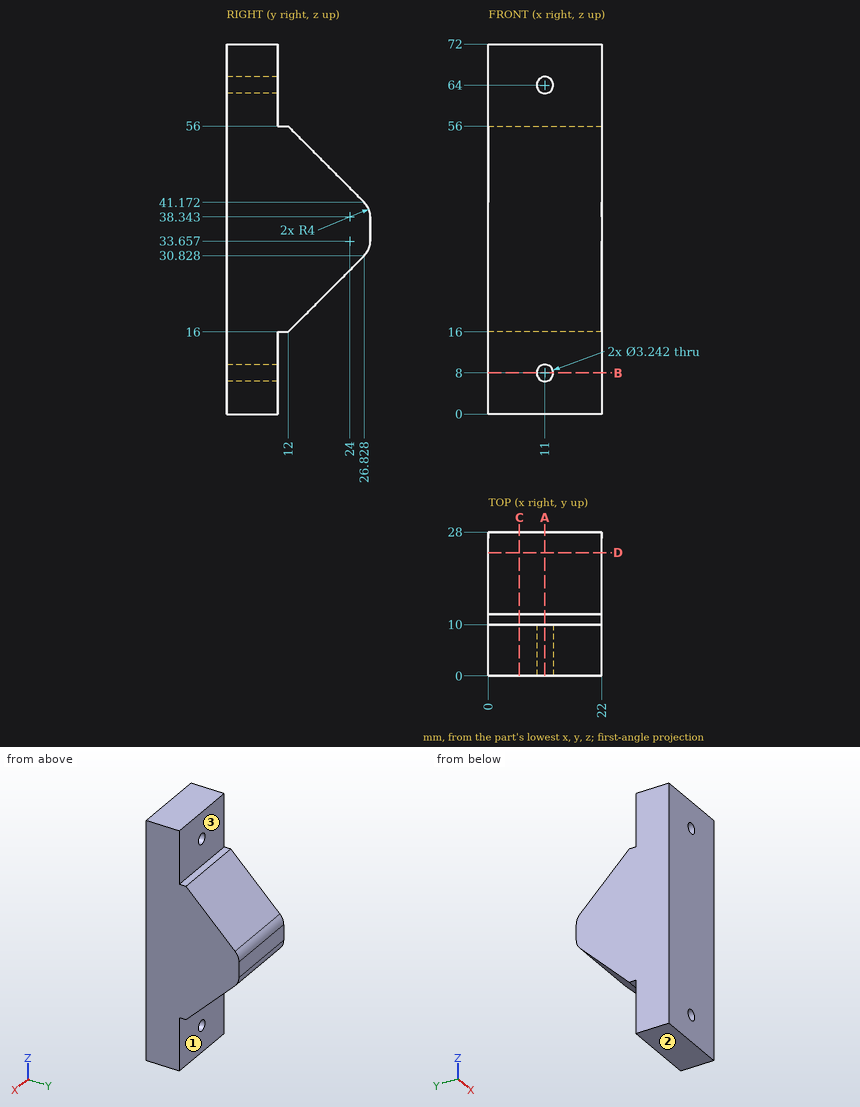
Answer from the drawing. Dimensions are ordinates in mm from the lowest x, y and z of the part. A direction names the side the tool comes from. Round coordinates to 2 decimals unless told otherwise and drop trailing zeros. Write each loop counter-clockwise with the first axis right and the second up, starting at its lowest first coordinate (ties: lowest second). Pieces come first, ordered by that corner, then holes. Notation, with made-up numbers: (-9, 78.5) - (9, 78.5) arc R16 cw to (9, 98.5) - close; hole circle Ø1 at (-32.5, 6.25). An arc over 180 degrees is marked (long way). One line per item, written item: value.
Q1. Find section D-D (y = 24). Determine the outline of the cut face in (x, z), and give its area (3 significant figures).
The answers:
outline: (0, 28) - (22, 28) - (22, 44) - (0, 44) - close
area: 352 mm2
Q2. Find section B-B (z = 8). Determine the outline of the cut face in (x, y).
The answers:
outline: (0, 0) - (9.38, 0) - (9.38, 10) - (0, 10) - close; (12.62, 0) - (22, 0) - (22, 10) - (12.62, 10) - close
Q3. Straight lines are drawn through the part: line 1 (Z direction, x = 11, y = 6.25); line 2 (X direction, y = 7, z = 64); line 3 (Y direction, x = 6.5, z = 12.5). For each, find the intervals that lie inside material, in ascending order. Write a range as from..to.
The answers:
line 1: z = 0..6.38, 9.62..62.38, 65.62..72
line 2: x = 0..9.38, 12.62..22
line 3: y = 0..10
Q4. Find section A-A (x = 11). Determine the outline of the cut face in (y, z).
The answers:
outline: (0, 0) - (10, 0) - (10, 6.38) - (0, 6.38) - close; (0, 9.62) - (10, 9.62) - (10, 16) - (12, 16) - (26.83, 30.83) arc R4 ccw to (28, 33.66) - (28, 38.34) arc R4 ccw to (26.83, 41.17) - (12, 56) - (10, 56) - (10, 62.38) - (0, 62.38) - close; (0, 65.62) - (10, 65.62) - (10, 72) - (0, 72) - close
Q5. Find section C-C (x = 6). Determine the outline of the cut face in (y, z).
The answers:
outline: (0, 0) - (10, 0) - (10, 16) - (12, 16) - (26.83, 30.83) arc R4 ccw to (28, 33.66) - (28, 38.34) arc R4 ccw to (26.83, 41.17) - (12, 56) - (10, 56) - (10, 72) - (0, 72) - close
Q6. Each of these flat-tipped pins is pushed along its axis until it touches: P1, Ø1, axis at x = 4, y = 24.5, coming from the -Z side; P2, Ø8, axis at x = 15, z = 8.5, coming from the +Y side; P3, Ø0.6, axis at x = 12, y = 11, coming from the -Z side. Where does it stop, or does it pass through?
The answers:
P1: stops at z = 28
P2: stops at y = 10
P3: stops at z = 16
Q7. Which of the six approach directions +Z, -Z, +X, -X, +Y, -Y give full straight-line access (tool end or side, diameter ignored) to the marked faces 1, 2 and 3?
The answers:
face 1: -Z, +X, -X, +Y
face 2: -Z, +X, -X, +Y, -Y
face 3: +Z, +X, -X, +Y
